Geometry: final body of the model. Coordinates: model frame, mm. A direction names the side the tool comes from. Coordinates: 2 decimals unless noted, no trailing zeros. Loops run counter-clockwise (first coordinate to the right, second up) from the corner with the lowest first, then second, coordinate; pieces in that order, holes last. Notation, with made-up numbers: M 25.5,11.5 L 73.5,11.5 A21 ccw 73.5,40.5 Z; hole C 7,-37.5 d8. An arc over 180 degrees is marked long. Write each question's results on one line, items separated by ' | '. Start each with the question number.
from build123d import *

# Parameters (mm, degrees)
F0_R     = 3.5
F1_DEPTH = 8
F2_R     = 1.75
F3_DEPTH = 12.001
F5_DEPTH = 5


with BuildPart() as f1:
    # F0 (on Front) → F1 (new body)
    with BuildSketch(Plane.XZ):
        with BuildLine():
            Line((-16, 1), (-16, 0))
            Line((-16, 0), (16, 0))
            Line((16, 0), (16, 1))
            ThreePointArc((16, 1), (15.414214, 2.414214), (14, 3))
            Line((14, 3), (8, 3))
            ThreePointArc((8, 3), (7.292893, 3.292893), (7, 4))
            Line((7, 4), (7, 5))
            ThreePointArc((7, 5), (4.949747, 9.949747), (0, 12))
            ThreePointArc((0, 12), (-4.949747, 9.949747), (-7, 5))
            Line((-7, 5), (-7, 4))
            ThreePointArc((-7, 4), (-7.292893, 3.292893), (-8, 3))
            Line((-8, 3), (-14, 3))
            ThreePointArc((-14, 3), (-15.414214, 2.414214), (-16, 1))
        make_face()
        with Locations((0, 5)):
            Circle(F0_R, mode=Mode.SUBTRACT)
    extrude(amount=F1_DEPTH)

    # F2 (on face) → F3 (cut, through all)
    with BuildSketch(Plane(origin=(0, 0, 0), x_dir=(1, 0, 0), z_dir=(0, 0, -1))):
        with Locations((-11, 4)):
            Circle(F2_R)
        with Locations((11, 4)):
            Circle(F2_R)
    extrude(amount=-F3_DEPTH, mode=Mode.SUBTRACT)

    # F4 (on face) → F5 (cut)
    with BuildSketch(Plane.XZ.offset(8)):
        with BuildLine():
            Line((5, 0), (5, 5))
            ThreePointArc((5, 5), (0, 10), (-5, 5))
            Line((-5, 5), (-5, 0))
            Line((-5, 0), (5, 0))
        make_face()
    extrude(amount=-F5_DEPTH, mode=Mode.SUBTRACT)


solid = f1.part
Item 1: Pull-direction query (Y, two-part tool) for faces 1 (the cylindrical face through (15.43, -3.94, 2.4)), 2 (the flat face through (3.3, 0, 3.4)), 3 (the cylindrical face through (-10.19, -2.45, 1.48)), 4 (the cylindrical face through (11.81, -2.45, 1.48)); classes: released by +Y, released by -Y, zero draft, split by the parting line, or undercut.
Item 2: Section D-D, the plane y = -6.5. Return loops of the section in (x, z), plus the area to 3 significant figures.
Item 3: Section A-A, the plane y = -4. Return loops of the section in (x, z).
Item 4: Ray query, L1, parallel to X at y = -1.3, z = 5; L2, parallel to X at y = -4, z = 0.9; L3, parallel to X at y = -4, z = 2.4. Return the intervals inside material, ascending. Write a range as [from, to].
Item 5: Set-up query: faces 5 (the flat face through (-2.3, -3, 1.7)), 6 (the flat face through (0, -2, 0)), 7 (the flat face through (7, -3.9, 4.5)), 8 (the flat face through (-11, -2, 3)). Return all of +Z, -Z, +X, -X, +Y, -Y with unobstructed straight access to the full face (end or side cutting, diameter ignored); none if empty.
Item 6: Contact query for flat-ended pins moving along their axis: P1, Ø2, axis at x = -7.5, y = -1, coming from the -Z side; P2, Ø0.8, axis at y = -3.5, z = 4.5, coming from the +X side; P3, Ø0.8, axis at y = -4.5, z = 4.5, coming from the -X side; P4, Ø1.5, axis at x = -5.5, y = -6.5, coming from the +Z side. Output: stop coordinate, or through.
Item 7: Section C-C, the plane x = 2. Return loops of the section in (y, z).
Item 8: Section B-B, the plane z = 7. Return loops of the section in (x, y).
Solutions:
1) face 1: zero draft | face 2: released by +Y | face 3: undercut | face 4: undercut
2) outline: M -16,0 L -5,0 L -5,5 A5 cw 5,5 L 5,0 L 16,0 L 16,1 A2 ccw 14,3 L 8,3 A1 cw 7,4 L 7,5 A7 ccw 0,12 A7 ccw -7,5 L -7,4 A1 cw -8,3 L -14,3 A2 ccw -16,1 Z | area: 110 mm²
3) outline: M -16,0 L -12.75,0 L -12.75,3 L -14,3 A2 ccw -16,1 Z; M -9.25,0 L -5,0 L -5,5 A5 cw 5,5 L 5,0 L 9.25,0 L 9.25,3 L 8,3 A1 cw 7,4 L 7,5 A7 ccw 0,12 A7 ccw -7,5 L -7,4 A1 cw -8,3 L -9.25,3 Z; M 12.75,0 L 16,0 L 16,1 A2 ccw 14,3 L 12.75,3 Z
4) L1: x = [-7, -3.5], [3.5, 7] | L2: x = [-16, -12.75], [-9.25, -5], [5, 9.25], [12.75, 16] | L3: x = [-15.43, -12.75], [-9.25, -5], [5, 9.25], [12.75, 15.43]
5) face 5: -Z, -Y | face 6: -Z, +X, -X, +Y, -Y | face 7: +Z, +X, +Y, -Y | face 8: +Z, -X, +Y, -Y
6) P1: stops at z = 0 | P2: stops at x = 7 | P3: stops at x = -7 | P4: stops at z = 10.14
7) outline: M -8,9.58 L -3,9.58 L -3,7.87 L 0,7.87 L 0,11.71 L -8,11.71 Z; M -3,0 L 0,0 L 0,2.13 L -3,2.13 Z
8) outline: M -6.71,-8 L -4.58,-8 L -4.58,-3 L -2.87,-3 L -2.87,0 L -6.71,0 Z; M 2.87,-3 L 4.58,-3 L 4.58,-8 L 6.71,-8 L 6.71,0 L 2.87,0 Z
